Here's how the part is built. I have some questions about the finished solid (model axes, mm). Face numbers are marked on the shaded views. A direction names the side the tool comes from. Give positions to 0.01 mm unless a question says otherwise; leave off trailing zeros. Order: outer loops, then holes, each group sorted by start corner. A loop starts at its lowest first (then second) coordinate and runs counter-clockwise, first axis right, second up. Notation, with made-up numbers: M -6,0.25 L 41,0.25 A17 ccw 41,8.25 Z; hole C 65.5,6 d7. An arc over 180 degrees is marked long. One line per item, written item: value. Start each with the question number.
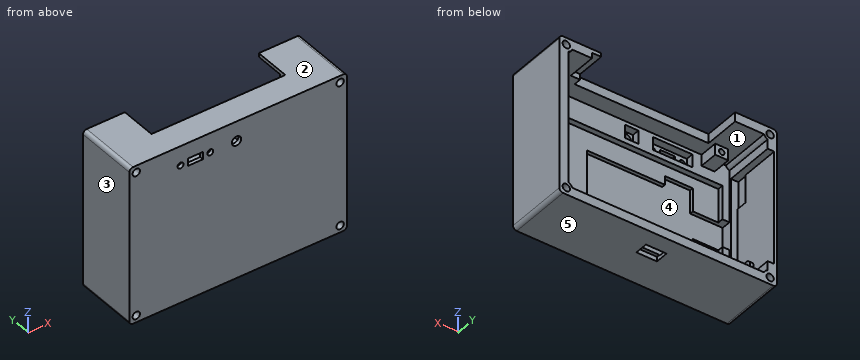
from build123d import *

# Parameters (mm, degrees)
SKETCH1_W                = 117
SKETCH1_H                = 85
BOSS_EXTRUDE1_DEPTH      = 34
SKETCH2_W                = 107
SKETCH2_H                = 75
CUT_EXTRUDE1_DEPTH       = 28
SKETCH3_R                = 2
CUT_EXTRUDE2_DEPTH       = 28
CUT_EXTRUDE2_DEPTH_BACK  = 28
SKETCH11_R               = 3.5
BOSS_EXTRUDE3_DEPTH      = 28
SKETCH13_R               = 2
CUT_EXTRUDE9_DEPTH       = 35
SKETCH14_W               = 102
SKETCH14_H               = 62
CUT_EXTRUDE10_DEPTH      = 3
SKETCH15_W               = 61
SKETCH15_H               = 40
CUT_EXTRUDE11_DEPTH      = 3.5
SKETCH16_W               = 15
SKETCH16_H               = 6
CUT_EXTRUDE12_DEPTH      = 0.5
CUT_EXTRUDE13_DEPTH      = 5
SKETCH20_W               = 72
SKETCH20_H               = 25
CUT_EXTRUDE14_DEPTH      = 5
SKETCH21_W               = 7
SKETCH21_H               = 2
CUT_EXTRUDE15_DEPTH      = 2
SKETCH22_W               = 7
SKETCH22_H               = 2
BOSS_EXTRUDE5_DEPTH      = 2.5
SKETCH23_W               = 3
SKETCH23_H               = 1.5
BOSS_EXTRUDE6_DEPTH      = 2.5
CUT_EXTRUDE17_DEPTH      = 92.5
SKETCH38_W               = 21
SKETCH38_H               = 7
CUT_EXTRUDE22_DEPTH      = 4
SKETCH39_R               = 1.6
SKETCH39_W               = 8
SKETCH39_H               = 4
CUT_EXTRUDE23_DEPTH      = 33
CUT_EXTRUDE23_DEPTH_BACK = 3
SKETCH40_W               = 7.2
SKETCH40_H               = 7.2
CUT_EXTRUDE24_DEPTH      = 4
SKETCH41_R               = 2.5
CUT_EXTRUDE25_DEPTH      = 4
FILLET5_R                = 2
FILLET6_R                = 2
FILLET7_R                = 2
FILLET8_R                = 2
SKETCH6_W                = 42
SKETCH6_H                = 30.5
CUT_EXTRUDE26_DEPTH      = 5
CUT_EXTRUDE27_DEPTH      = 5
CUT_EXTRUDE27_DEPTH_BACK = 2
SKETCH43_R               = 3
SKETCH43_R_2             = 1.5
BOSS_EXTRUDE7_DEPTH      = 2
SKETCH44_W               = 5
SKETCH44_H               = 15.5
CUT_EXTRUDE28_DEPTH      = 3
SKETCH45_W               = 18
SKETCH45_H               = 2.5
CUT_EXTRUDE29_DEPTH      = 3
SKETCH47_W               = 11.05
SKETCH47_H               = 7
CUT_EXTRUDE30_DEPTH      = 2.5
SKETCH48_W               = 7
SKETCH48_H               = 6
BOSS_EXTRUDE8_DEPTH      = 10
SKETCH49_W               = 7
SKETCH49_H               = 6
BOSS_EXTRUDE9_DEPTH      = 10
SKETCH51_R               = 1.5
CUT_EXTRUDE31_DEPTH      = 8
SKETCH50_R               = 1.5
CUT_EXTRUDE32_DEPTH      = 8


with BuildPart() as part:
    # Sketch1 → Boss-Extrude1 (new body)
    with BuildSketch(Plane(origin=(0, 0, 0), x_dir=(1, 0, 0), z_dir=(0, 1, 0))):
        Rectangle(SKETCH1_W, SKETCH1_H)
    extrude(amount=BOSS_EXTRUDE1_DEPTH)

    # Sketch2 → Cut-Extrude1 (cut)
    with BuildSketch(Plane(origin=(0, 34, 0), x_dir=(1, 0, 0), z_dir=(0, 1, 0))):
        Rectangle(SKETCH2_W, SKETCH2_H)
    extrude(amount=-CUT_EXTRUDE1_DEPTH, mode=Mode.SUBTRACT)

    # Sketch3 → Cut-Extrude2 (cut, two sides)
    with BuildSketch(Plane(origin=(0, 6, 0), x_dir=(1, 0, 0), z_dir=(0, 1, 0))) as cut_extrude2_sk:
        with Locations((54.8, -38.8)):
            Circle(SKETCH3_R)
        with Locations((54.8, 38.8)):
            Circle(SKETCH3_R)
        with Locations((-54.8, 38.8)):
            Circle(SKETCH3_R)
        with Locations((-54.8, -38.8)):
            Circle(SKETCH3_R)
    extrude(amount=CUT_EXTRUDE2_DEPTH, mode=Mode.SUBTRACT)
    extrude(cut_extrude2_sk.sketch, amount=-CUT_EXTRUDE2_DEPTH_BACK, mode=Mode.SUBTRACT)

    # Sketch11 → Boss-Extrude3 (add)
    with BuildSketch(Plane(origin=(0, 6, 0), x_dir=(1, 0, 0), z_dir=(0, 1, 0))):
        with Locations((-54.8, -38.8)):
            Circle(SKETCH11_R)
        with Locations((-54.8, 38.8)):
            Circle(SKETCH11_R)
        with Locations((54.8, -38.8)):
            Circle(SKETCH11_R)
        with Locations((54.8, 38.8)):
            Circle(SKETCH11_R)
    extrude(amount=BOSS_EXTRUDE3_DEPTH)

    # Sketch13 → Cut-Extrude9 (cut, through all)
    with BuildSketch(Plane(origin=(0, 34, 0), x_dir=(1, 0, 0), z_dir=(0, 1, 0))):
        with Locations((-54.8, 38.8)):
            Circle(SKETCH13_R)
        with Locations((54.8, 38.8)):
            Circle(SKETCH13_R)
        with Locations((-54.8, -38.8)):
            Circle(SKETCH13_R)
        with Locations((54.8, -38.8)):
            Circle(SKETCH13_R)
    extrude(amount=-CUT_EXTRUDE9_DEPTH, mode=Mode.SUBTRACT)

    # Sketch14 → Cut-Extrude10 (cut)
    with BuildSketch(Plane(origin=(0, 6, 0), x_dir=(1, 0, 0), z_dir=(0, 1, 0))):
        with Locations((1.3, 5.3)):
            Rectangle(SKETCH14_W, SKETCH14_H)
    extrude(amount=-CUT_EXTRUDE10_DEPTH, mode=Mode.SUBTRACT)

    # Sketch15 → Cut-Extrude11 (cut)
    with BuildSketch(Plane(origin=(-53.5, 0, 0), x_dir=(0, 0, -1), z_dir=(1, 0, 0))):
        with Locations((-0.000384638, 27)):
            Rectangle(SKETCH15_W, SKETCH15_H)
    extrude(amount=-CUT_EXTRUDE11_DEPTH, mode=Mode.SUBTRACT)

    # Sketch16 → Cut-Extrude12 (cut)
    with BuildSketch(Plane(origin=(-57, 0, 0), x_dir=(0, 0, -1), z_dir=(1, 0, 0))):
        with Locations((-23.000384638, 10)):
            Rectangle(SKETCH16_W, SKETCH16_H)
    extrude(amount=-CUT_EXTRUDE12_DEPTH, mode=Mode.SUBTRACT)

    # Sketch18 → Cut-Extrude13 (cut)
    with BuildSketch(Plane(origin=(0, 0, -42.5), x_dir=(-1, 0, 0), z_dir=(0, 0, -1))):
        with BuildLine():
            Line((-3.725, 23.5), (3.725, 23.5))
            ThreePointArc((3.725, 23.5), (5.475, 21.75), (3.725, 20))
            Line((3.725, 20), (-3.725, 20))
            ThreePointArc((-3.725, 20), (-5.475, 21.75), (-3.725, 23.5))
        make_face()
    extrude(amount=-CUT_EXTRUDE13_DEPTH, mode=Mode.SUBTRACT)

    # Sketch20 → Cut-Extrude14 (cut)
    with BuildSketch(Plane.XY.offset(42.5)):
        with Locations((0, 27)):
            Rectangle(SKETCH20_W, SKETCH20_H)
    extrude(amount=-CUT_EXTRUDE14_DEPTH, mode=Mode.SUBTRACT)

    # Sketch21 → Cut-Extrude15 (cut)
    with BuildSketch(Plane.XY.offset(-37.5)):
        with Locations((-41.050384638, 17)):
            Rectangle(SKETCH21_W, SKETCH21_H)
        with Locations((41.050384638, 17)):
            Rectangle(SKETCH21_W, SKETCH21_H)
    extrude(amount=-CUT_EXTRUDE15_DEPTH, mode=Mode.SUBTRACT)

    # Sketch22 → Boss-Extrude5 (add)
    with BuildSketch(Plane(origin=(0, 0, 37.5), x_dir=(-1, 0, 0), z_dir=(0, 0, -1))):
        with Locations((-43.800384638, 15)):
            Rectangle(SKETCH22_W, SKETCH22_H)
        with Locations((41.990384638, 15)):
            Rectangle(SKETCH22_W, SKETCH22_H)
    extrude(amount=BOSS_EXTRUDE5_DEPTH)

    # Sketch23 → Boss-Extrude6 (add)
    with BuildSketch(Plane(origin=(0, 0, 37.5), x_dir=(-1, 0, 0), z_dir=(0, 0, -1))):
        with Locations((-43.800384638, 13.25)):
            Rectangle(SKETCH23_W, SKETCH23_H)
        with Locations((43.800384638, 13.25)):
            Rectangle(SKETCH23_W, SKETCH23_H)
    extrude(amount=BOSS_EXTRUDE6_DEPTH)

    # Sketch25 → Cut-Extrude17 (cut)
    with BuildSketch(Plane(origin=(45.300384638, 0, 0), x_dir=(0, 0, -1), z_dir=(1, 0, 0))):
        Polygon((-35, 14), (-37.5, 12.5), (-35, 12.5), align=None)
    extrude(amount=-CUT_EXTRUDE17_DEPTH, mode=Mode.SUBTRACT)

    # Sketch38 → Cut-Extrude22 (cut)
    with BuildSketch(Plane(origin=(0, 6, 0), x_dir=(1, 0, 0), z_dir=(0, 1, 0))):
        with Locations((-23, -32)):
            Rectangle(SKETCH38_W, SKETCH38_H)
    extrude(amount=-CUT_EXTRUDE22_DEPTH, mode=Mode.SUBTRACT)

    # Sketch39 → Cut-Extrude23 (cut, two sides)
    with BuildSketch(Plane(origin=(0, 2, 0), x_dir=(1, 0, 0), z_dir=(0, 1, 0))) as cut_extrude23_sk:
        with Locations((-31, -32)):
            Circle(SKETCH39_R)
        with Locations((-15, -32)):
            Circle(SKETCH39_R)
        with Locations((-23, -32)):
            Rectangle(SKETCH39_W, SKETCH39_H)
    extrude(amount=CUT_EXTRUDE23_DEPTH, mode=Mode.SUBTRACT)
    extrude(cut_extrude23_sk.sketch, amount=-CUT_EXTRUDE23_DEPTH_BACK, mode=Mode.SUBTRACT)

    # Sketch40 → Cut-Extrude24 (cut)
    with BuildSketch(Plane(origin=(0, 6, 0), x_dir=(1, 0, 0), z_dir=(0, 1, 0))):
        with Locations((-0.9, -31.9)):
            Rectangle(SKETCH40_W, SKETCH40_H)
    extrude(amount=-CUT_EXTRUDE24_DEPTH, mode=Mode.SUBTRACT)

    # Sketch41 → Cut-Extrude25 (cut)
    with BuildSketch(Plane(origin=(0, 2, 0), x_dir=(1, 0, 0), z_dir=(0, 1, 0))):
        with Locations((-0.9, -31.9)):
            Circle(SKETCH41_R)
    extrude(amount=-CUT_EXTRUDE25_DEPTH, mode=Mode.SUBTRACT)

    # Fillet5
    fillet5_edges = [part.edges().sort_by_distance(p)[0] for p in [
        (-58.5, 17, 42.5),
    ]]
    fillet(fillet5_edges, radius=FILLET5_R)

    # Fillet6
    fillet6_edges = [part.edges().sort_by_distance(p)[0] for p in [
        (58.5, 17, 42.5),
    ]]
    fillet(fillet6_edges, radius=FILLET6_R)

    # Fillet7
    fillet7_edges = [part.edges().sort_by_distance(p)[0] for p in [
        (58.5, 17, -42.5),
    ]]
    fillet(fillet7_edges, radius=FILLET7_R)

    # Fillet8
    fillet8_edges = [part.edges().sort_by_distance(p)[0] for p in [
        (-58.5, 17, -42.5),
    ]]
    fillet(fillet8_edges, radius=FILLET8_R)

    # Sketch6 → Cut-Extrude26 (cut)
    with BuildSketch(Plane(origin=(22.627458043, 6, 6.502354234), x_dir=(1, 0, 0), z_dir=(0, 1, 0))):
        with Locations((-22.627458043, 6.502354234)):
            Rectangle(SKETCH6_W, SKETCH6_H)
    extrude(amount=-CUT_EXTRUDE26_DEPTH, mode=Mode.SUBTRACT)

    # Sketch42 → Cut-Extrude27 (cut, two sides)
    with BuildSketch(Plane(origin=(0, 3, 0), x_dir=(1, 0, 0), z_dir=(0, 1, 0))) as cut_extrude27_sk:
        Polygon((-21, -20), (-36, -20), (-36, -7.5), (-53.5, -7.5), (-53.5, 7.5), (-36, 7.5), (-36, 20), (-21, 20), align=None)
    extrude(amount=CUT_EXTRUDE27_DEPTH, mode=Mode.SUBTRACT)
    extrude(cut_extrude27_sk.sketch, amount=-CUT_EXTRUDE27_DEPTH_BACK, mode=Mode.SUBTRACT)

    # Sketch43 → Boss-Extrude7 (add)
    with BuildSketch(Plane(origin=(-57, 0, 0), x_dir=(0, 0, -1), z_dir=(1, 0, 0))):
        with Locations((22.499615362, 16)):
            Circle(SKETCH43_R)
        with Locations((22.499615362, 16)):
            Circle(SKETCH43_R_2, mode=Mode.SUBTRACT)
    extrude(amount=BOSS_EXTRUDE7_DEPTH)

    # Sketch44 → Cut-Extrude28 (cut)
    with BuildSketch(Plane(origin=(0, 0, 37.5), x_dir=(-1, 0, 0), z_dir=(0, 0, -1))):
        with Locations((-38.5, 26.25)):
            Rectangle(SKETCH44_W, SKETCH44_H)
    extrude(amount=-CUT_EXTRUDE28_DEPTH, mode=Mode.SUBTRACT)

    # Sketch45 → Cut-Extrude29 (cut)
    with BuildSketch(Plane.XY.offset(-37.5)):
        with Locations((0, 21.25)):
            Rectangle(SKETCH45_W, SKETCH45_H)
    extrude(amount=-CUT_EXTRUDE29_DEPTH, mode=Mode.SUBTRACT)

    # Sketch47 → Cut-Extrude30 (cut)
    with BuildSketch(Plane(origin=(0, 0, -42.5), x_dir=(-1, 0, 0), z_dir=(0, 0, -1))):
        with Locations((0, 21.75)):
            Rectangle(SKETCH47_W, SKETCH47_H)
    extrude(amount=-CUT_EXTRUDE30_DEPTH, mode=Mode.SUBTRACT)

    # Sketch48 → Boss-Extrude8 (add)
    with BuildSketch(Plane(origin=(0, 16, 0), x_dir=(1, 0, 0), z_dir=(0, 1, 0))):
        with Locations((43.800384638, -34.5)):
            Rectangle(SKETCH48_W, SKETCH48_H)
    extrude(amount=-BOSS_EXTRUDE8_DEPTH)

    # Sketch49 → Boss-Extrude9 (add)
    with BuildSketch(Plane(origin=(0, 16, 0), x_dir=(1, 0, 0), z_dir=(0, 1, 0))):
        with Locations((-41.990384638, -34.5)):
            Rectangle(SKETCH49_W, SKETCH49_H)
    extrude(amount=-BOSS_EXTRUDE9_DEPTH)

    # Sketch51 → Cut-Extrude31 (cut)
    with BuildSketch(Plane(origin=(0, 16, 0), x_dir=(1, 0, 0), z_dir=(0, 1, 0))):
        with Locations((-41.985384638, -34.5)):
            Circle(SKETCH51_R)
    extrude(amount=-CUT_EXTRUDE31_DEPTH, mode=Mode.SUBTRACT)

    # Sketch50 → Cut-Extrude32 (cut)
    with BuildSketch(Plane(origin=(0, 16, 0), x_dir=(1, 0, 0), z_dir=(0, 1, 0))):
        with Locations((43.795384638, -34.5)):
            Circle(SKETCH50_R)
    extrude(amount=-CUT_EXTRUDE32_DEPTH, mode=Mode.SUBTRACT)


solid = part.part
Item 1: For the marked faces 1 and 2, which set-ups out of +Z, -Z, +X, -X, +Y, -Y let a thin tool reach every point of the face, with its end or its side?
Item 2: I want a section at B-B on x = -31. Write out the boundary of the cut face in (y, z).
Item 3: I want a section at D-D on z = 1. Write out the boundary of the cut face in (x, y), plus the area to 3 significant figures.
Item 4: I want a section at C-C on z = 38.8. Write out the boundary of the cut face in (x, y), plus the area to 3 significant figures.
Item 5: Will these pins go through, and if not, where does the flat tip stop? P1, Ø4, axis at x = 18, z = -30.5, coming from the -Y side; P2, Ø3, axis at x = 54.8, z = 38.8, coming from the -Y side; P3, Ø20, axis at x = -5, z = 6.5, coming from the +Y side; P4, Ø6, axis at x = -36.5, z = 26.5, coming from the +Y side.
Item 6: We'd pull the mould along X, two halves only. Please class the marked faces 3, 4 and 5: +X half, -X half, draft (parallel to the pull), parting line (faces both ways), or undercut.
Item 7: Please list where these lines run through material, in increasing order: probe 1 along X at (y, z) = (10, 34.5); probe 2 along Z at (x, y) = (-54.8, 14); probe 3 along X at (y, z) = (19, 38.8). Write a range as [from, to].
Item 8: I want a section at A-A on x = -0.9. Count the separate pieces of the cut face and the enclosed holes in it, plus the area to 3 significant figures.
Answer below:
1. face 1: +Y
1. face 2: +Z, +X, -X, +Y, -Y
2. outline: M 0,-42.5 L 34,-42.5 L 34,-37.5 L 6,-37.5 L 6,-36.3 L 3,-36.3 L 3,-20 L 1,-20 L 1,20 L 3,20 L 3,25.7 L 6,25.7 L 6,28.5 L 2,28.5 L 2,30.4 L 0,30.4 Z; M 0,33.6 L 2,33.6 L 2,35.5 L 6,35.5 L 6,37.5 L 14.5,37.5 L 14.5,42.5 L 0,42.5 Z
3. outline: M -58.5,0 L 58.5,0 L 58.5,34 L 53.5,34 L 53.5,6 L 52.3,6 L 52.3,3 L 21,3 L 21,1 L -53.5,1 L -53.5,7 L -57,7 L -57,34 L -58.5,34 Z
3. area: 421 mm²
4. outline: M -58.5,0 L -56.8,0 L -56.8,34 L -58.5,34 Z; M -52.8,0 L 52.8,0 L 52.8,34 L 41,34 L 41,18.5 L 36,18.5 L 36,14.5 L -36,14.5 L -36,34 L -52.8,34 Z; M 56.8,0 L 58.5,0 L 58.5,34 L 56.8,34 Z
4. area: 2,220 mm²
5. P1: stops at y = 0
5. P2: passes through
5. P3: stops at y = 3
5. P4: stops at y = 6
6. face 3: -X half
6. face 4: undercut
6. face 5: draft
7. probe 1: x = [-58.5, -53.5], [-45.49, -43.49], [-40.49, -38.49], [40.3, 42.3], [45.3, 47.3], [53.5, 58.5]
7. probe 2: z = [-42.5, -40.8], [-36.8, -30.5], [30.5, 36.8], [40.8, 42.5]
7. probe 3: x = [-58.5, -56.8], [-52.8, -36], [41, 52.8], [56.8, 58.5]
8. separate pieces: 3
8. enclosed holes: 0
8. area: 380 mm²
